Autodesk Inventor part; units mm, degrees
ref_plane "YZ Plane" through (0, 0, 0) normal (1, 0, 0) x (0, 1, 0)
ref_plane "XZ Plane" through (0, 0, 0) normal (0, 1, 0) x (-1, 0, 0)
ref_plane "XY Plane" through (0, 0, 0) normal (0, 0, 1) x (1, 0, 0)
sketch "Sketch1" plane through (0, 0, 0) normal (0, 1, 0) x (-1, 0, 0)
  circle A0 centre (0, 0) radius 11.915
  circle A1 centre (0, 0) radius 9.8
  circle A2 centre (0, 0) radius 8.25
  circle A3 centre (0, 0) radius 6.5
  circle A4 centre (6.5, 0) radius 0.65
  circle A5 centre (9.8, 0) radius 0.65
  circle A6 centre (9.054, 3.7503) radius 0.65
  circle A7 centre (6.0052, 2.4874) radius 0.65
  circle A8 centre (9.054, -3.7503) radius 0.65
  circle A9 centre (6.0052, -2.4874) radius 0.65
  circle A10 centre (-9.054, -3.7503) radius 0.65
  circle A11 centre (-6.0052, -2.4874) radius 0.65
  circle A12 centre (-6.5, 0) radius 0.65
  circle A13 centre (-9.8, 0) radius 0.65
  circle A14 centre (-6.0052, 2.4874) radius 0.65
  circle A15 centre (-9.054, 3.7503) radius 0.65
  circle A16 centre (0, 8.25) radius 0.65
  circle A17 centre (-3.1571, 7.622) radius 0.65
  circle A18 centre (3.1571, 7.622) radius 0.65
  circle A19 centre (-3.1571, -7.622) radius 0.65
  circle A20 centre (0, -8.25) radius 0.65
  circle A21 centre (3.1571, -7.622) radius 0.65
  circle A22 centre (0, 0) radius 1.37
  circle A23 centre (0, 0) radius 2.75
  circle A24 centre (0, 0) radius 2.97
  circle A25 centre (0, 0) radius 3.73
  circle A26 centre (0, 0) radius 4.44
  dimension "d1" = 19.6
  dimension "d2" = 16.5
  dimension "d3" = 13
  dimension "d0" = 23.83
  dimension "d4" = 1.3
  dimension "d5" = 1.3
  dimension "d8" = 22.5
  dimension "d12" = 337.5
  dimension "d16" = 180
  dimension "d18" = 1.3
  dimension "d21" = 22.5
  dimension "d25" = 337.5
  dimension "d29" = 180
  dimension "d31" = 2.74
  dimension "d32" = 5.5
  dimension "d33" = 5.94
  dimension "d34" = 7.46
  dimension "d35" = 8.88
extrude "Extrusion1" add sketch "Sketch1" along normal blind 2 contours A0 | A5 A1 A8 A10 A13 A15 A6 | A2 A21 A20 A19 A17 A16 A18 | A4 A3 A9 A11 A12 A14 A7
extrude "Extrusion2" add sketch "Sketch1" along normal blind 4.5 contours A26
extrude "Extrusion3" add sketch "Sketch1" along normal blind 4.5 and the other way blind 0.5 contours A25
extrude "Extrusion4" add sketch "Sketch1" along normal blind 4.5 contours A24
extrude "Extrusion5" add sketch "Sketch1" along normal blind 0.75 contours A23
properties part number "Standard Servo Horn - White Circle"
The listing builds one solid part. Answer for the finished solid, in the listing's coordinates (mm). A direction names the side the tool comes from. Coordinates: 2 decimals unless noted, no trailing zeros. Write each loop counter-clockwise with the first axis right and the second up, starting at its lowest first coordinate (ties: lowest second). Pieces come first, ordered by that corner, then holes.
Q1. Find the intervals of material crossed by line 1 along Z through (x, y) = (0, 0.7) (3 decimals); line 2 along X through (y, z) = (1.8, -4); line 3 along Z through (x, y) = (-6.5, 0.6), in increasing order.
Returned:
line 1: z = -11.915 to -8.9, -7.6 to -1.37, 1.37 to 7.6, 8.9 to 11.915
line 2: x = -11.22 to -9.65, -8.45 to 8.45, 9.65 to 11.22
line 3: z = -9.99 to -2.91, -2.07 to -0.65, 0.65 to 2.07, 2.91 to 9.99
Q2. Given P1, Ø2, axis at x = -7.5, z = 9.5, coming from the +Y side; P2, Ø1.5, axis at x = -9.05, z = -3.75, coming from the -Y side; P3, Ø1, axis at x = -9.05, z = 3.75, coming from the +Y side; P4, Ø1, axis at y = 1, z = 1.5, coming from the +X side, each flat-ended and moving along its own axis, determine where each tip first touches the part or whether it passes through.
Returned:
P1: stops at y = 2
P2: stops at y = 0
P3: passes through
P4: stops at x = 11.87
Q3. Section D-D, the plane y = 4.1 is taken. Write down the section's boundary in (x, z), then the cut area to 3 significant figures.
Returned:
outline: circle Ø8.88 at (0, 0); hole circle Ø5.5 at (0, 0)
area: 38.2 mm2
Q4. Section A-A, the plane x = 0 is taken. Give the number of separate pieces and of enclosed holes in the cut face, then the cut area to 3 significant figures.
Returned:
separate pieces: 4
enclosed holes: 0
area: 42.7 mm2
Q5. Section B-B, the plane z = -1 is taken. Write down the section's boundary in (x, y), then the cut area to 3 significant figures.
Returned:
outline: (-11.87, 0) - (-3.59, 0) - (-3.59, -0.5) - (-2.8, -0.5) - (-2.8, 0) - (-0.94, 0) - (-0.94, 0.75) - (-2.56, 0.75) - (-2.56, 4.5) - (-4.33, 4.5) - (-4.33, 2) - (-11.87, 2) - close; (0.94, 0) - (2.8, 0) - (2.8, -0.5) - (3.59, -0.5) - (3.59, 0) - (11.87, 0) - (11.87, 2) - (4.33, 2) - (4.33, 4.5) - (2.56, 4.5) - (2.56, 0.75) - (0.94, 0.75) - close
area: 49.3 mm2
Q6. The mould has two halves that part along Z. Classify faces 1 (the cylindrical face through (0.963, 3.232, 4.334)), 2 (the flat face through (3, 0, 3)), 3 (the cylindrical face through (-6.625, 0.986, 2.292)): released by +Z, released by -Z, zero draft, split by the parting line, or undercut.
Returned:
face 1: split by the parting line
face 2: zero draft
face 3: undercut
Q7. Which of the six approach directions +Z, -Z, +X, -X, +Y, -Y give full straight-line access (tool end or side, diameter ignored) to faces 4 (the cylindrical face through (6.09, 0.986, 1.843)), 5 (the flat face through (-5, 2, 0))?
Returned:
face 4: +Y, -Y
face 5: +Y
